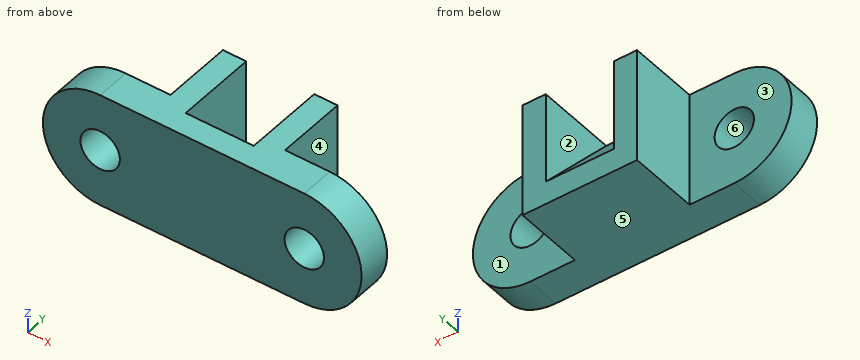
from build123d import *

# Parameters (mm, degrees)
SKETCH1_R               = 11
BOSS_EXTRUDE1_DEPTH     = 13
SKETCH2_W               = 38
SKETCH2_H               = 51
BOSS_EXTRUDE3_DEPTH     = 45
CUT_EXTRUDE1_DEPTH      = 127.696487718
CUT_EXTRUDE1_DEPTH_BACK = 127.696487718
SKETCH4_R               = 11
BOSS_EXTRUDE4_DEPTH     = 6
BOSS_EXTRUDE5_DEPTH     = 39


with BuildPart() as part:
    # Sketch1 → Boss-Extrude1 (new body)
    with BuildSketch(Plane(origin=(0, 0, 0), x_dir=(1, 0, 0), z_dir=(0, 1, 0))):
        with BuildLine():
            Line((-57, 32), (57, 32))
            ThreePointArc((57, 32), (89, 0), (57, -32))
            Line((57, -32), (-57, -32))
            ThreePointArc((-57, -32), (-89, 0), (-57, 32))
        make_face()
        with Locations(Location((-57, 0, 0), (0, 0, 90))):
            Circle(SKETCH1_R, mode=Mode.SUBTRACT)
        with Locations(Location((57, 0, 0), (0, 0, 90))):
            Circle(SKETCH1_R, mode=Mode.SUBTRACT)
    extrude(amount=BOSS_EXTRUDE1_DEPTH)

    # Sketch2 → Boss-Extrude3 (add)
    with BuildSketch(Plane(origin=(0, 13, 0), x_dir=(1, 0, 0), z_dir=(0, 1, 0))):
        with Locations((0, -6.5)):
            Rectangle(SKETCH2_W, SKETCH2_H)
    extrude(amount=BOSS_EXTRUDE3_DEPTH)

    # Sketch3 → Cut-Extrude1 (cut, two sides: drawn at the far end of the back side and taken through both)
    with BuildSketch(Plane.ZY.offset(19).offset(-CUT_EXTRUDE1_DEPTH_BACK)):
        Polygon((-143.828237157, 168.142562197), (-19, 58), (32, 13), (156.828237157, -97.142562197), (377.113361551, 152.513912116), (76.456887238, 417.799036511), align=None)
    extrude(amount=CUT_EXTRUDE1_DEPTH + CUT_EXTRUDE1_DEPTH_BACK, mode=Mode.SUBTRACT)

    # Sketch4 → Boss-Extrude4 (add)
    with BuildSketch(Plane(origin=(0, 13, 0), x_dir=(1, 0, 0), z_dir=(0, 1, 0))):
        with BuildLine():
            ThreePointArc((-57, 32), (-89, 0), (-57, -32))
            Line((-57, -32), (-19, -32))
            Line((-19, -32), (-19, 19))
            Line((-19, 19), (19, 19))
            Line((19, 19), (19, -32))
            Line((19, -32), (57, -32))
            ThreePointArc((57, -32), (89, 0), (57, 32))
            Line((57, 32), (-57, 32))
        make_face()
        with Locations(Location((-57, 0, 0), (0, 0, 90))):
            Circle(SKETCH4_R, mode=Mode.SUBTRACT)
        with Locations(Location((57, 0, 0), (0, 0, 90))):
            Circle(SKETCH4_R, mode=Mode.SUBTRACT)
    extrude(amount=BOSS_EXTRUDE4_DEPTH)

    # Sketch5 → Boss-Extrude5 (add)
    with BuildSketch(Plane(origin=(0, 19, 0), x_dir=(1, 0, 0), z_dir=(0, 1, 0))):
        Polygon((-32, 32), (32, 32), (32, -32), (19, -32), (19, -25.2), (19, 19), (-19, 19), (-19, -25.2), (-19, -32), (-32, -32), align=None)
    extrude(amount=BOSS_EXTRUDE5_DEPTH)


solid = part.part
Could you check a few things on this model? Use its own coordinates, in mm. Face numbers are marked on the shaded views. A direction names the side the tool comes from. Round coordinates to 2 decimals unless told otherwise and drop trailing zeros. Loops run counter-clockwise (first coordinate to the right, second up) from the corner with the lowest first, then second, coordinate; pieces in that order, holes last. Notation, with made-up numbers: (74.25, 24) - (116.25, 24) arc R21 cw to (116.25, 44) - close; hole circle Ø10 at (-38.75, 60.25). An arc over 180 degrees is marked (long way). Write item = value, one per line.
1) Imagine slicing it at C-C (y = 46). Please give me the cut outline in (x, z).
Computed:
outline = (-32, -32) - (32, -32) - (32, 32) - (19, 32) - (19, -5.4) - (-19, -5.4) - (-19, 32) - (-32, 32) - close
2) Imagine slicing it at D-D (x = 41). Please give me the cut outline in (y, z), and give its area (3 significant figures).
Computed:
outline = (0, -32) - (19, -32) - (19, 32) - (0, 32) - close
area = 1,220 mm2
3) Imagine slicing it at B-B (z = 0). Please give me the cut outline in (x, y).
Computed:
outline = (-89, 0) - (-68, 0) - (-68, 19) - (-89, 19) - close; (-46, 0) - (46, 0) - (46, 19) - (32, 19) - (32, 58) - (19, 58) - (19, 41.24) - (-19, 41.24) - (-19, 58) - (-32, 58) - (-32, 19) - (-46, 19) - close; (68, 0) - (89, 0) - (89, 19) - (68, 19) - close
4) On a 3-axis mill with a long thin cutter (end or side, diameter ignored), from which of +Z, -Z, +X, -X, +Y, -Y can I reach the whole of each face in a straight line? I mean the marked faces 1, 2 and 3. Say none if no direction works.
Computed:
face_1 = +Z, -Z, +X, +Y
face_2 = +Z, +Y
face_3 = +Z, -Z, -X, +Y
5) I'm going to push flat-ended pins straight in: P1, Ø5, axis at x = 65, y = 11, coming from the +Z side; P2, Ø17.5, axis at x = 57, z = 0, coming from the -Y side; P3, Ø6, axis at y = 8.5, z = -23, coming from the -X side; P4, Ø4, axis at y = 47.5, z = -4.5, coming from the +X side. Where does each tip first touch, or does it pass through?
Computed:
P1 = 31.52
P2 = through
P3 = -81.98
P4 = 32
6) Imagine slicing it at A-A (x = 59). Please give me the cut outline in (y, z).
Computed:
outline = (0, -31.94) - (19, -31.94) - (19, -10.82) - (0, -10.82) - close; (0, 10.82) - (19, 10.82) - (19, 31.94) - (0, 31.94) - close
7) If we mould it in two halves opening along Z, with no side actions, what happens to the marked faces 4, 5 and 6? For each: pulls with the +Z half, pulls with the -Z half, needs draft (parallel to the pull), parting line crosses it, or undercut.
Computed:
face_4 = needs draft
face_5 = pulls with the -Z half
face_6 = undercut
8) I need wall thicknesses on line 1 along X through (y, z) = (11, 0); line 2 along X through (y, z) = (48, 17); line 3 along Z through (x, y) = (57, 10). Which ranges of each line are inside material? Lowest first, please. Write a range as from..to.
Computed:
line_1 = -89..-68, -46..46, 68..89
line_2 = -32..-19, 19..32
line_3 = -32..-11, 11..32
